Check sheet for the modelled part. Datum: model origin and axes. Units: mm. Coordinates: 2 decimals unless noted, no trailing zeros. Write each loop counter-clockwise with the first axis right and the second up, starting at its lowest first coordinate (ties: lowest second). Pieces come first, ordered by that corner, then holes. Notation, with made-up numbers: (-4.75, 78.5) -> (42.25, 78.5) arc R28 ccw to (42.25, 101.5) -> close; hole circle Ø8 at (23, -40). An arc over 180 degrees is marked (long way). One line per item, written item: value. Start each with the question number.
1) Sectioned sample at C-C on z = 4. Enter the section's corners in (x, y).
2) Scan lines: line 1 along X through (y, z) = (30.55, -5.5); line 2 along Z through (x, y) = (31, 30.35); line 3 along Z through (x, y) = (11, 30.3). Record each from-to range of solid material in increasing order. Write a range as [from, to].
3) Sectioned sample at D-D on y = 30.6. Give the number of separate pieces and of enclosed holes in the cut face, plus the area to 3 significant figures.
4) Sectioned sample at B-B on x = 32. Enter the section's corners in (y, z).
5) Sectioned sample at A-A on x = 46.5. Enter the section's corners in (y, z), plus the area to 3 significant figures.
6) Gauge pin test, flat ends, axial feed: P1, Ø0.5, axis at y = 30.5, z = 81, coming from the -X side; P2, Ø0.5, axis at x = 48, y = 30.5, coming from the -Z side; P3, Ø0.5, axis at x = 11, y = 30.5, coming from the +Z side; P4, Ø4, axis at x = -0.81, z = 96.09, coming from the +Y side. Record the tip position at first contact, or that the pin passes through.
```python
from build123d import *

# Parameters (mm, degrees)
COVER_MAIN_BOARD_1_START = 30
COVER_MAIN_BOARD_1_DEPTH = 1
SKETCH_2_R               = 2.5
SKETCH_2_R_2             = 3
EXTRUDE_1_DEPTH          = 1
FILLET_1_R               = 6
HOLE_WIZARD_M31_D        = 3.2
SKETCH_5_W               = 20
SKETCH_5_H               = 13
CUT_EXTRUDE_2_DEPTH      = 118.861812366
FILLET_2_R               = 2
SKETCH_7_W               = 10
SKETCH_7_H               = 4
SKETCH_7_W_2             = 9
CUT_EXTRUDE_4_DEPTH      = 118.861812366
FILLET_3_R               = 1.5
CUT_EXTRUDE_5_DEPTH      = 118.861812366


# Read off the part's stored shape, not the designer's step: Припуск-Cover_main_board-1
with BuildPart() as part:
    # Припуск-Cover_main_board-1 outline → Припуск-Cover_main_board-1 (new body)
    with BuildSketch(Plane(origin=(0, 0, 0), x_dir=(1, 0, 0), z_dir=(0, 1, 0)).offset(COVER_MAIN_BOARD_1_START)):
        with BuildLine():
            ThreePointArc((58.536662962, -97.610509717), (61.872887908, -97.542255565), (62.936422695, -94.379353532))
            add(Edge.make_bspline(
                [(62.936422695, -94.379353532), (61.798177223, -90.776493028), (60.72075986, -87.155811957), (58.774674414, -79.85329338), (57.908149184, -76.177190929), (56.466060339, -68.758031881), (55.893308454, -65.032046108), (55.109773151, -57.544971093), (54.899999704, -53.783069267), (54.9, -50)],
                knots=[0, 0, 0, 0, 0.25, 0.25, 0.5, 0.5, 0.75, 0.75, 1, 1, 1, 1], degree=3))
            Line((54.9, -50), (54.9, 6.4))
            Line((54.9, 6.4), (5.1, 6.4))
            Line((5.1, 6.4), (5.1, -50))
            add(Edge.make_bspline(
                [(5.1, -50), (5.099991031, -53.776486453), (4.890826579, -57.541590974), (4.10432522, -65.051764617), (3.53002006, -68.780548712), (2.088476888, -76.191600122), (1.222062078, -79.86132679), (-0.718312327, -87.143485068), (-1.7924779, -90.75713228), (-2.928662588, -94.354417399)],
                knots=[0, 0, 0, 0, 0.25, 0.25, 0.5, 0.5, 0.75, 0.75, 1, 1, 1, 1], degree=3))
            ThreePointArc((-2.928662588, -94.354417399), (-1.883263044, -97.534459074), (1.463338472, -97.610508751))
            ThreePointArc((1.463338472, -97.610508751), (30.000000864, -88.89999981), (58.536662962, -97.610509717))
        make_face()
    extrude(amount=COVER_MAIN_BOARD_1_DEPTH)

    # Эскиз2 → Бобышка-Вытянуть1 (add)
    with BuildSketch(Plane(origin=(0, 31, 0), x_dir=(1, 0, 0), z_dir=(0, 1, 0))):
        with Locations((6, 5.5)):
            Circle(SKETCH_2_R)
        with Locations((54, 5.5)):
            Circle(SKETCH_2_R)
        with Locations((-0.811267397, -96.088490424)):
            Circle(SKETCH_2_R_2)
        with Locations((60.811267397, -96.088490424)):
            Circle(SKETCH_2_R_2)
    extrude(amount=-EXTRUDE_1_DEPTH)

    # Скругление1
    fillet_1_edges = [part.edges().sort_by_distance(p)[0] for p in [
        (-2.75519034, 30.5, 93.803503862),
        (1.934506666, 30.5, 97.297094907),
        (58.065493335, 30.5, 97.297094908),
        (62.755023846, 30.5, 93.803362229),
        (54.9, 30.5, -3.167619242),
        (51.667619242, 30.5, -6.4),
        (8.332380758, 30.5, -6.4),
        (5.1, 30.5, -3.167619242),
    ]]
    fillet(fillet_1_edges, radius=FILLET_1_R)

    # Отверстие с зазором M31 (through all)
    with Locations(Plane(origin=(0, 31, 0), x_dir=(1, 0, 0), z_dir=(0, 1, 0))):
        with Locations((-0.811267397, -96.088490424), (60.811267397, -96.088490424), (54, 5.5), (6, 5.5)):
            Hole(HOLE_WIZARD_M31_D / 2)

    # Эскиз5 → Вырез-Вытянуть2 (cut, through all)
    with BuildSketch(Plane.XZ.offset(-30)):
        with Locations((30, 80.64999981)):
            Rectangle(SKETCH_5_W, SKETCH_5_H)
    extrude(amount=-CUT_EXTRUDE_2_DEPTH, mode=Mode.SUBTRACT)

    # Скругление2
    fillet_2_edges = [part.edges().sort_by_distance(p)[0] for p in [
        (40, 30.5, 87.14999981),
        (40, 30.5, 74.14999981),
        (20, 30.5, 74.14999981),
        (20, 30.5, 87.14999981),
    ]]
    fillet(fillet_2_edges, radius=FILLET_2_R)

    # Эскиз7 → Вырез-Вытянуть4 (cut, through all)
    with BuildSketch(Plane.XZ.offset(-30)):
        with Locations((47.9, 80.6)):
            Rectangle(SKETCH_7_W, SKETCH_7_H)
        with Locations((12.6, 80.6)):
            Rectangle(SKETCH_7_W_2, SKETCH_7_H)
    extrude(amount=-CUT_EXTRUDE_4_DEPTH, mode=Mode.SUBTRACT)

    # Скругление3
    fillet_3_edges = [part.edges().sort_by_distance(p)[0] for p in [
        (42.9, 30.5, 78.6),
        (42.9, 30.5, 82.6),
        (52.9, 30.5, 82.6),
        (52.9, 30.5, 78.6),
        (17.1, 30.5, 82.6),
        (17.1, 30.5, 78.6),
        (8.1, 30.5, 78.6),
        (8.1, 30.5, 82.6),
    ]]
    fillet(fillet_3_edges, radius=FILLET_3_R)

    # Эскиз10 → Вырез-Вытянуть5 (cut, through all)
    with BuildSketch(Plane(origin=(0, 31, 0), x_dir=(1, 0, 0), z_dir=(0, 1, 0))):
        with BuildLine():
            Line((42.9, -80.1), (52.9, -80.1))
            Line((52.9, -80.1), (52.9, -78.1))
            ThreePointArc((52.9, -78.1), (52.460660172, -77.039339828), (51.4, -76.6))
            Line((51.4, -76.6), (44.4, -76.6))
            ThreePointArc((44.4, -76.6), (43.339339828, -77.039339828), (42.9, -78.1))
            Line((42.9, -78.1), (42.9, -80.1))
        make_face()
        with BuildLine():
            Line((8.1, -80.1), (17.1, -80.1))
            Line((17.1, -80.1), (17.1, -78.1))
            ThreePointArc((17.1, -78.1), (16.660660172, -77.039339828), (15.6, -76.6))
            Line((15.6, -76.6), (9.6, -76.6))
            ThreePointArc((9.6, -76.6), (8.539339828, -77.039339828), (8.1, -78.1))
            Line((8.1, -78.1), (8.1, -80.1))
        make_face()
    extrude(amount=-CUT_EXTRUDE_5_DEPTH, mode=Mode.SUBTRACT)


solid = part.part
```
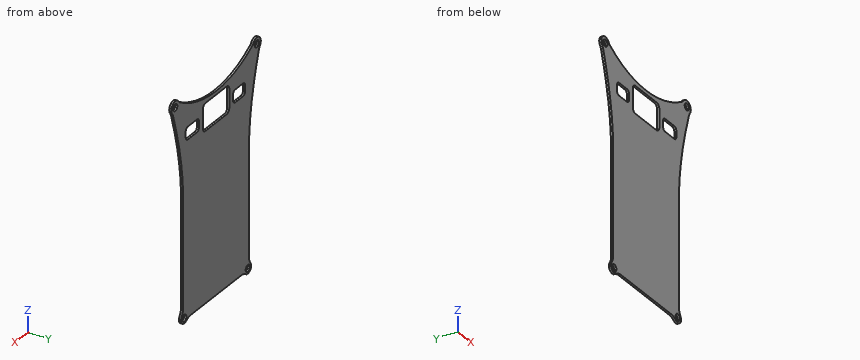
Answers:
1. outline: (5.1, 30) -> (54.9, 30) -> (54.9, 31) -> (5.1, 31) -> close
2. line 1: x = [3.5, 4.4], [7.6, 52.4], [55.6, 56.5]
2. line 2: z = [-6.4, 74.15], [87.15, 88.91]
2. line 3: z = [-6.4, 76.6], [82.6, 92.56]
3. separate pieces: 1
3. enclosed holes: 7
3. area: 4,780 mm2
4. outline: (30, -6.4) -> (31, -6.4) -> (31, 74.15) -> (30, 74.15) -> close; (30, 87.15) -> (31, 87.15) -> (31, 88.94) -> (30, 88.94) -> close
5. outline: (30, -6.4) -> (31, -6.4) -> (31, 76.6) -> (30, 76.6) -> close; (30, 82.6) -> (31, 82.6) -> (31, 91.64) -> (30, 91.64) -> close
5. area: 92.0 mm2
6. P1: stops at x = 0.84
6. P2: stops at z = -6.4
6. P3: stops at z = 92.66
6. P4: stops at y = 31
